Design review of the part shown in the three views and the two pictorial views. Dimensions are in mm from the part's minimum x, y and z. A direction names the side the tool comes from. Coordinates: 2 decimals unless noted, no trailing zeros. Order: outer loops, then holes, each group sorted by start corner. A loop starts at its lowest first (then second) coordinate and runs counter-clockwise, first axis right, second up. Notation, with made-up numbers: (83.25, 22) -> (108.25, 22) arc R23 cw to (108.25, 48) -> close; hole circle Ø11 at (18, 66). An arc over 180 degrees is marked (long way). Answer as a JSON object with one key per item and string values. Group by question number.
1) Wall thickness on L1, parallel to Z at x = 2.15, y = 2.85; L2, parallel to X at y = 4.2, z = 2.1; L3, parallel to X at y = 2.3, z = 0.9: over which ranges is each line inside the solid? List them lowest first.
2) Add section D-D, the plane x = 4.6. Write out the cut boundary in (y, z), then the cut area to 3 significant figures.
3) Add section C-C, the plane x = 0.65. Write out the cut boundary in (y, z), then the cut area to 3 significant figures.
4) Machinability: for the marked faces 1 and 2, which of the approach directions +Z, -Z, +X, -X, +Y, -Y give a long, thin tool a straight path to every point of the face, cutting with its end or side? Answer none if there is none.
5) For pin 1 (1 mm diameter, centred on x = 2.5, y = 1, fed in from +Z); pin 2 (3 mm diameter, centred on x = 3, y = 0.5, fed in from +Z); pin 3 (1 mm diameter, centred on y = 5, z = 0.5, fed in from -X), all flat-tipped, find the tip position at first contact; note any pin that passes through.
6) Add section A-A, the plane z = 2.85. Write out the cut boundary in (x, y).
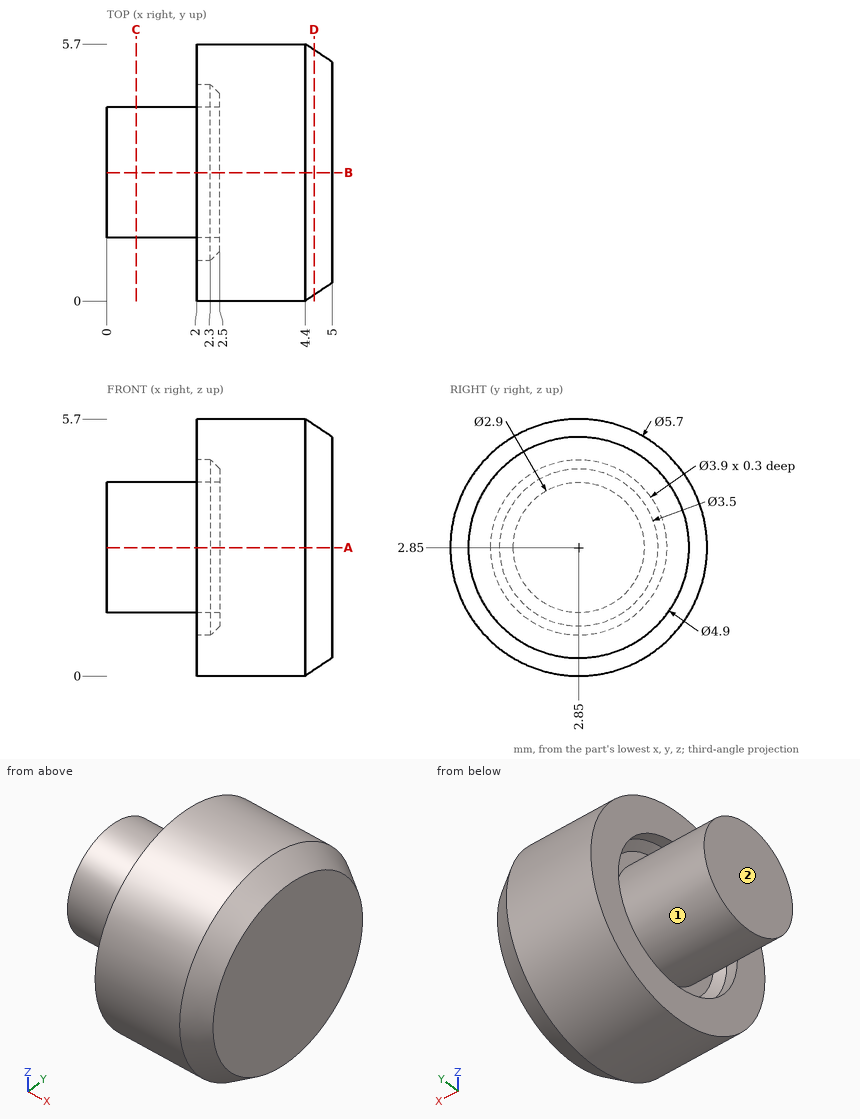
Output values:
{
 "1": {"L1": "z = 0 to 0.9, 1.4 to 4.3, 4.8 to 5.7", "L2": "x = 2.5 to 5", "L3": "x = 2 to 5"},
 "2": {"outline": "circle Ø5.43 at (2.85, 2.85)", "area": "23.2 mm²"},
 "3": {"outline": "circle Ø2.9 at (2.85, 2.85)", "area": "6.61 mm²"},
 "4": {"face 1": "-X", "face 2": "+Z, -Z, -X, +Y, -Y"},
 "5": {"pin 1": "stops at z = 5.36", "pin 2": "stops at z = 5.57", "pin 3": "stops at x = 2"},
 "6": {"outline": "(0, 1.4) -> (2.5, 1.4) -> (2.5, 1.1) -> (2.3, 0.9) -> (2, 0.9) -> (2, 0) -> (4.4, 0) -> (5, 0.4) -> (5, 5.3) -> (4.4, 5.7) -> (2, 5.7) -> (2, 4.8) -> (2.3, 4.8) -> (2.5, 4.6) -> (2.5, 4.3) -> (0, 4.3) -> close"}
}
